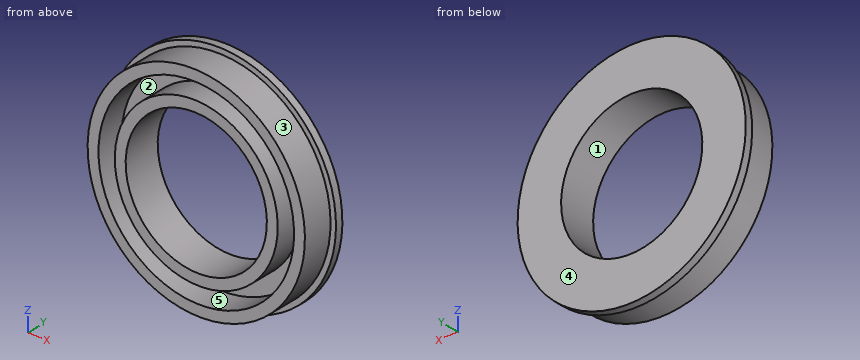
from build123d import *

# Parameters (mm, degrees)
ESQUISSE1_R      = 10
ESQUISSE1_R_2    = 6.5
EXTRUSION1_DEPTH = 3.5
ESQUISSE2_R      = 10.5
ESQUISSE2_R_2    = 10
EXTRUSION2_DEPTH = 0.7
COQUE1_T         = -1


with BuildPart() as part:
    # Esquisse1 → Extrusion1 (new body)
    with BuildSketch(Plane(origin=(0, 0, 0), x_dir=(1, 0, 0), z_dir=(0, 1, 0))):
        with Locations(Location((0, 0, 0), (0, 0, 270))):  # turned: the seam where the file's is
            Circle(ESQUISSE1_R)
        with Locations(Location((0, 0, 0), (0, 0, 270))):  # turned: the seam where the file's is
            Circle(ESQUISSE1_R_2, mode=Mode.SUBTRACT)
    extrude(amount=-EXTRUSION1_DEPTH)

    # Esquisse2 → Extrusion2 (add)
    with BuildSketch(Plane(origin=(0, 0, 0), x_dir=(-1, 0, 0), z_dir=(0, 1, 0))):
        with Locations(Location((0, 0, 0), (0, 0, 90))):  # turned: the seam where the file's is
            Circle(ESQUISSE2_R)
        with Locations(Location((0, 0, 0), (0, 0, 90))):  # turned: the seam where the file's is
            Circle(ESQUISSE2_R_2, mode=Mode.SUBTRACT)
    extrude(amount=-EXTRUSION2_DEPTH)

    # Coque1
    coque1_openings = [part.faces().sort_by_distance(p)[0] for p in [
        (0, -3.5, -9.717157288),
    ]]
    offset(amount=COQUE1_T, openings=coque1_openings, kind=Kind.INTERSECTION)


solid = part.part
Can you work these out from the model? Positions are in its coordinate system, mm. Face numbers are marked on the shaded views. A direction names the side the tool comes from. Coordinates: 2 decimals unless noted, no trailing zeros. Loops run counter-clockwise (first coordinate to the right, second up) from the corner with the lowest first, then second, coordinate; pieces in that order, holes last. Notation, with made-up numbers: (78, 73.5) - (91, 73.5) arc R18 ccw to (91, 104.5) - close; hole circle Ø3 at (-14.75, 73.5). An arc over 180 degrees is marked (long way). Put each result on its own line as item: value. Start each with the question number.
Item 1: If we mould it in two halves opening along X, with no side actions, what happens to the marked faces 3, 4 and 5? For each: +X half, -X half, draft (parallel to the pull), parting line (faces both ways), or undercut.
Item 2: Suppose I cut it at A-A (x = 0). Please give me the cut outline in (y, z).
Item 3: Suppose I cut it at D-D (x = 7). Please give me the cut outline in (y, z), and give its area (3 significant figures).
Item 4: Which directions (+Z, -Z, +X, -X, +Y, -Y) give clear straight access to the entire face, cutting with the end or side of a thin tool? Please do the marked faces 1 and 2.
Item 5: If I drill on line 1 along X through (y, z) = (-1.45, 0); line 2 along Z through (x, y) = (-2.5, -1.75); line 3 along X through (y, z) = (-2.65, -5.25), over which ranges is the centre line in solid material (lowest first)?
Item 6: For pin 1 (1.5 mm diameter, centred on y = -2, z = 1, fed in from +X); pin 2 (1.5 mm diameter, centred on x = -6, y = -3, fed in from -Z); pin 3 (1.5 mm diameter, centred on y = -3, z = 2, fed in from -X), each with a flat end and sliding along its axis, tell me the tip position at first contact or that it passes through.
Item 7: Suppose I cut it at B-B (y = -2.85). Please give me the cut outline in (x, z).
Item 8: Suppose I cut it at C-C (z = 0). Please give me the cut outline in (x, y).
Here are the results:
1. face 3: parting line
1. face 4: draft
1. face 5: undercut
2. outline: (-3.5, -10) - (-0.7, -10) - (-0.7, -10.5) - (0, -10.5) - (0, -6.5) - (-3.5, -6.5) - (-3.5, -7.5) - (-1, -7.5) - (-1, -9) - (-3.5, -9) - close; (-3.5, 6.5) - (0, 6.5) - (0, 10.5) - (-0.7, 10.5) - (-0.7, 10) - (-3.5, 10) - (-3.5, 9) - (-1, 9) - (-1, 7.5) - (-3.5, 7.5) - close
3. outline: (-3.5, -7.14) - (-0.7, -7.14) - (-0.7, -7.83) - (0, -7.83) - (0, 7.83) - (-0.7, 7.83) - (-0.7, 7.14) - (-3.5, 7.14) - (-3.5, 5.66) - (-1, 5.66) - (-1, 2.69) - (-3.5, 2.69) - (-3.5, -2.69) - (-1, -2.69) - (-1, -5.66) - (-3.5, -5.66) - close
3. area: 36.1 mm²
4. face 1: +Y, -Y
4. face 2: -Y
5. line 1: -10 to -9, -7.5 to -6.5, 6.5 to 7.5, 9 to 10
5. line 2: -9.68 to -8.65, -7.07 to -6, 6 to 7.07, 8.65 to 9.68
5. line 3: -8.51 to -7.31, -5.36 to -3.83, 3.83 to 5.36, 7.31 to 8.51
6. pin 1: x = 10
6. pin 2: z = -8.51
6. pin 3: x = -9.92
7. outline: circle Ø20 at (0, 0); circle Ø15 at (0, 0); hole circle Ø18 at (0, 0); hole circle Ø13 at (0, 0)
8. outline: (-10.5, -0.7) - (-10, -0.7) - (-10, -3.5) - (-9, -3.5) - (-9, -1) - (-7.5, -1) - (-7.5, -3.5) - (-6.5, -3.5) - (-6.5, 0) - (-10.5, 0) - close; (6.5, -3.5) - (7.5, -3.5) - (7.5, -1) - (9, -1) - (9, -3.5) - (10, -3.5) - (10, -0.7) - (10.5, -0.7) - (10.5, 0) - (6.5, 0) - close
